Check sheet for the modelled part. Datum: model origin and axes. Units: mm. Face numbers are marked on the shaded views. A direction names the side the tool comes from. Round coordinates to 2 decimals unless told otherwise and drop trailing zeros. Order: outer loops, then holes, each group sorted by start corner. A loop starts at its lowest first (then second) coordinate and runs counter-clockwise, first axis right, second up. Notation, with made-up numbers: (25.5, 30) -> (67.5, 30) arc R6 ccw to (67.5, 38) -> close; hole circle Ø9 at (-6, 0). An arc over 180 degrees is marked (long way). Answer in a Markdown table with one row per item.
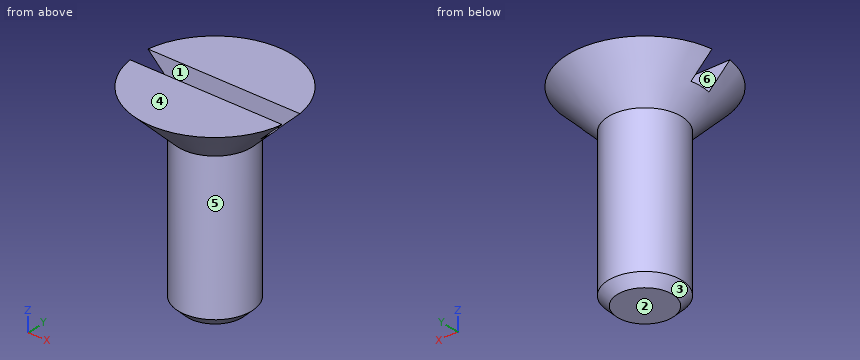
```python
from build123d import *

# Parameters (mm, degrees)
SKETCH9_W          = 6.3
SKETCH9_H          = 0.875
CUT_EXTRUDE1_DEPTH = 0.85


with BuildPart() as part:
    # Sketch3 → Revolve1 (revolve)
    with BuildSketch(Plane(origin=(0, 0, 0), x_dir=(0, 0, -1), z_dir=(1, 0, 0)), mode=Mode.PRIVATE) as revolve1_sk:
        Polygon((-1.7, 3.15), (-0.05, 1.5), (5.925, 1.5), (6.3, 1.125), (6.3, 0), (-1.7, 0), align=None)
    revolve(revolve1_sk.sketch.rotate(Axis((0, 0, 1.7), (0, 0, -1)), 90), axis=Axis((0, 0, 1.7), (0, 0, -1)))

    # Sketch9 → Cut-Extrude1 (cut)
    with BuildSketch(Plane.XY.offset(1.7)):
        Rectangle(SKETCH9_W, SKETCH9_H)
    extrude(amount=-CUT_EXTRUDE1_DEPTH, mode=Mode.SUBTRACT)


solid = part.part
```
(1) Section check B-B on y = 0. Record the boundary of the cut face in (x, z) (3 decimals), plus the area to 3 significant figures.
Solutions:
| item | result |
|---|---|
| outline | (-2.3, 0.85) -> (-1.5, 0.05) -> (-1.5, -5.925) -> (-1.125, -6.3) -> (1.125, -6.3) -> (1.5, -5.925) -> (1.5, 0.05) -> (2.3, 0.85) -> close |
| area | 21.9 mm^2 |
(2) Depth check by flat-ended pin: pin 1 Ø3 at (x, z) = (0.5, -2.5) entering from -Y; pin 2 Ø0.9 at (x, z) = (-0.5, 1.5) entering from -Y; pin 3 Ø3 at (x, z) = (1.5, -1.5) entering from +Y; pin 4 Ø3 at (y, z) = (0, 0.5) entering from -X. Enter the tip coordinate at first touch or a pass-through.
Solutions:
| item | result |
|---|---|
| pin 1 | y = -1.5 |
| pin 2 | y = -3.15 |
| pin 3 | y = 1.5 |
| pin 4 | x = -3.12 |
(3) Draft check along Y on the marked faces 1, 2 and 3. Enter one of: pulls with the +Y half, pulls with the -Y half, needs draft (parallel to the pull), parting line crosses it, or undercut.
Solutions:
| item | result |
|---|---|
| face 1 | undercut |
| face 2 | needs draft |
| face 3 | parting line crosses it |
(4) Section check C-C on z = -3.5. Record the boundary of the cut face in (x, y), plus the area to 3 significant figures.
Solutions:
| item | result |
|---|---|
| outline | circle Ø3 at (0, 0) |
| area | 7.07 mm^2 |
(5) Tool access check on the marked faces 4, 5 and 6. Record the directions out of +Z, -Z, +X, -X, +Y, -Y that give a thin tool (end or side, any length) a straight path to the whole face; none if there is none.
Solutions:
| item | result |
|---|---|
| face 4 | +Z, +X, -X, +Y, -Y |
| face 5 | -Z |
| face 6 | +Z, +X, -X |
(6) Scan lines: probe 1 along Z at (x, y) = (-0.5, 2); probe 2 along X at (y, z) = (0.5, 0.5); probe 3 along X at (y, z) = (-0.75, -2.5). Record each from-to range of solid material in increasing order. Write a range as from..to.
Solutions:
| item | result |
|---|---|
| probe 1 | 0.61..1.7 |
| probe 2 | -1.88..1.88 |
| probe 3 | -1.3..1.3 |
